Geometry check sheet. Reference: the model listing, model coordinates, mm. A direction names the side the tool comes from. Coordinates: 2 decimals unless noted, no trailing zeros. Loops run counter-clockwise (first coordinate to the right, second up) from the corner with the lowest first, then second, coordinate; pieces in that order, holes last.
from build123d import *

# Parameters (mm, degrees)
SKETCH1_R           = 1.5
BOSS_EXTRUDE1_DEPTH = 2
SKETCH2_R           = 1.5
BOSS_EXTRUDE2_DEPTH = 3
BOSS_EXTRUDE3_DEPTH = 6
BOSS_EXTRUDE4_DEPTH = 2
CUT_EXTRUDE1_DEPTH  = 2
CUT_EXTRUDE2_DEPTH  = 4
BOSS_EXTRUDE5_DEPTH = 2


with BuildPart() as part:
    # Sketch1 → Boss-Extrude1 (new body)
    with BuildSketch(Plane.XY):
        with BuildLine():
            Line((-6.244997998, 5), (6.244997998, 5))
            ThreePointArc((6.244997998, 5), (8, 0), (6.244997998, -5))
            Line((6.244997998, -5), (-6.244997998, -5))
            ThreePointArc((-6.244997998, -5), (-8, 0), (-6.244997998, 5))
        make_face()
        Circle(SKETCH1_R, mode=Mode.SUBTRACT)
    extrude(amount=BOSS_EXTRUDE1_DEPTH)

    # Sketch2 → Boss-Extrude2 (add)
    with BuildSketch(Plane.XY.offset(2)):
        with BuildLine():
            Line((-4.898979486, -5), (4.898979486, -5))
            ThreePointArc((4.898979486, -5), (7, 0), (4.898979486, 5))
            Line((4.898979486, 5), (-4.898979486, 5))
            ThreePointArc((-4.898979486, 5), (-7, 0), (-4.898979486, -5))
        make_face()
        Circle(SKETCH2_R, mode=Mode.SUBTRACT)
    extrude(amount=BOSS_EXTRUDE2_DEPTH)

    # Sketch3 → Boss-Extrude3 (add)
    with BuildSketch(Plane(origin=(0, 0, 0), x_dir=(-1, 0, 0), z_dir=(0, 0, -1))):
        with BuildLine():
            Line((-6.244997998, -5), (-9.244997998, -5))
            ThreePointArc((-9.244997998, -5), (-10.584743961, 0), (-9.244997998, 5))
            Line((-9.244997998, 5), (-6.244997998, 5))
            ThreePointArc((-6.244997998, 5), (-8, 0), (-6.244997998, -5))
        make_face()
    extrude(amount=-BOSS_EXTRUDE3_DEPTH)

    # Sketch4 → Boss-Extrude4 (add)
    with BuildSketch(Plane.XY.offset(6)):
        with BuildLine():
            Line((7.416198487, 3), (10.124135975, 3))
            ThreePointArc((10.124135975, 3), (10.584743961, 0), (10.124135975, -3))
            Line((10.124135975, -3), (7.416198487, -3))
            ThreePointArc((7.416198487, -3), (8, 0), (7.416198487, 3))
        make_face()
    extrude(amount=BOSS_EXTRUDE4_DEPTH)

    # Sketch5 → Cut-Extrude1 (cut)
    with BuildSketch(Plane.XY.offset(5)):
        with BuildLine():
            Line((-1.5, 5), (-1.5, 0))
            ThreePointArc((-1.5, 0), (-4.1e-08, -1.5), (1.5, -8.1e-08))
            Line((1.5, -8.1e-08), (1.5, 5))
            Line((1.5, 5), (-1.5, 5))
        make_face()
    extrude(amount=-CUT_EXTRUDE1_DEPTH, mode=Mode.SUBTRACT)

    # Sketch6 → Cut-Extrude2 (cut)
    with BuildSketch(Plane.XY.offset(3)):
        with BuildLine():
            Line((-1.5, 5), (1.5, 5))
            Line((1.5, 5), (1.5, 3.995198361))
            ThreePointArc((1.5, 3.995198361), (0, 2.495198361), (-1.5, 3.995198361))
            Line((-1.5, 3.995198361), (-1.5, 5))
        make_face()
    extrude(amount=-CUT_EXTRUDE2_DEPTH, mode=Mode.SUBTRACT)

    # Sketch7 → Boss-Extrude5 (add)
    with BuildSketch(Plane.XY.offset(2)):
        with BuildLine():
            Line((4.898979486, -5), (6.244997998, -5))
            ThreePointArc((6.244997998, -5), (8, 0), (6.244997998, 5))
            Line((6.244997998, 5), (4.898979486, 5))
            ThreePointArc((4.898979486, 5), (7, 0), (4.898979486, -5))
        make_face()
    extrude(amount=BOSS_EXTRUDE5_DEPTH)


solid = part.part
(1) Draft check along X on faces 6 (the cylindrical face through (-7, 0, 3)), 7 (the flat face through (1, -5, 3)), 8 (the flat face through (0, 2, 3)). Enter one of: +X half, -X half, draft (parallel to the pull), parting line (faces both ways), or undercut.
Findings:
face 6: -X half
face 7: draft
face 8: undercut
(2) Sectioned sample at B-B on x = 0. Record the cut outline in (y, z), and give its area (3 significant figures).
Findings:
outline: (-5, 0) - (-1.5, 0) - (-1.5, 5) - (-5, 5) - close; (1.5, 0) - (2.5, 0) - (2.5, 3) - (1.5, 3) - close
area: 20.5 mm2
(3) Gauge pin test, flat ends, axial feed: pin 1 Ø0.6 at (x, y) = (7.5, -4) entering from +Z; pin 2 Ø2.5 at (x, y) = (-7, -2.5) entering from +Z; pin 3 Ø1.5 at (y, z) = (3, 3) entering from -X. Record the tip position at first contact, or that the pin passes through.
Findings:
pin 1: stops at z = 6
pin 2: stops at z = 5
pin 3: stops at x = -6.63
(4) Sectioned sample at D-D on z = 2.25. Record the cut outline in (x, y) (3 decimals).
Findings:
outline: (-4.899, -5) - (9.245, -5) arc R10 ccw to (9.245, 5) - (1.5, 5) - (1.5, 3.995) arc R1.5 cw to (-1.5, 3.995) - (-1.5, 5) - (-4.899, 5) arc R7 ccw to start; hole circle Ø3 at (0, 0)
(5) Access from +Z, -Z, +X, -X, +Y, -Y to the whole of each face (thin tool, end or side, straight path). Record for faces 1 (the flat face through (8, -4, 6)), 2 (the flat face through (8, 4, 6)), 3 (the flat face through (1.5, 3, 4)), 4 (the flat face through (7.2, -0.3, 4)), 5 (the flat face through (-7.2, -0.3, 2)).
Findings:
face 1: +Z, +X, -X, -Y
face 2: +Z, +X, -X, +Y
face 3: +Z, +Y
face 4: +Z
face 5: +Z, -X
(6) Sectioned sample at C-C on y = -1. Record the cut outline in (x, z).
Findings:
outline: (-7.94, 0) - (-1.12, 0) - (-1.12, 5) - (-6.93, 5) - (-6.93, 2) - (-7.94, 2) - close; (1.12, 0) - (10.53, 0) - (10.53, 8) - (7.94, 8) - (7.94, 4) - (6.93, 4) - (6.93, 5) - (1.12, 5) - close
(7) Sectioned sample at A-A on z = 4.75. Record the cut outline in (x, y) (3 decimals), and give its area (4 significant figures).
Findings:
outline: (-4.899, -5) - (4.899, -5) arc R7 ccw to (4.899, 5) - (1.5, 5) - (1.5, 0) arc R1.5 cw to (-1.5, 0) - (-1.5, 5) - (-4.899, 5) arc R7 ccw to start; (6.245, -5) - (9.245, -5) arc R10 ccw to (9.245, 5) - (6.245, 5) arc R8 cw to start
area: 135.5 mm2
(8) Scan lines: L1, parallel to Y at x = 0, z = 2.2; L2, parallel to Z at x = 5.75, y = 2.25; L3, parallel to Y at x = 1, z = 0.5. Record each from-to range of solid material in increasing order.
Findings:
L1: y = -5 to -1.5, 1.5 to 2.5
L2: z = 0 to 5
L3: y = -5 to -1.12, 1.12 to 2.88
